```python
from build123d import *

# Parameters (mm, degrees)
F1_DEPTH = 63.5
F0_W     = 25.4
F0_H     = 19.05
F2_DEPTH = 25.4
F3_DEPTH = 7.9375
F5_R     = 6.35


with BuildPart() as f1:
    # F0 (on Front) → F1 (new body, symmetric)
    with BuildSketch(Plane.XZ):
        Polygon((-41.275, -9.525), (41.275, -9.525), (41.275, 9.525), (22.225, 9.525), (-41.275, 9.525), align=None)
    extrude(amount=F1_DEPTH, both=True)



with BuildPart() as f2:
    # F0 (on Front) → F2 (new body, symmetric)
    with BuildSketch(Plane.XZ):
        with BuildLine():
            Line((22.225, 9.525), (41.275, 9.525))
            Line((41.275, 9.525), (41.275, 26.9875))
            ThreePointArc((41.275, 26.9875), (45.9246798487, 38.2128201513), (57.15, 42.8625))
            Line((57.15, 42.8625), (60.325, 42.8625))
            Line((60.325, 42.8625), (60.325, 61.9125))
            Line((60.325, 61.9125), (57.15, 61.9125))
            add(Edge.make_bspline(
                [(56.2230819512, 61.9001975172), (56.5320743429, 61.9050863843), (56.8410510368, 61.9091866589), (57.15, 61.9125)],
                knots=[110.7034248849, 110.7034248849, 110.7034248849, 110.7034248849, 111.4985685166, 111.4985685166, 111.4985685166, 111.4985685166], degree=3))
            ThreePointArc((56.2230819512, 61.9001975172), (32.1287266725, 51.3532855624), (22.225, 26.9875))
            Line((22.225, 26.9875), (22.225, 9.525))
        make_face()
        with Locations((73.025, 52.3875)):
            Rectangle(F0_W, F0_H)
    extrude(amount=F2_DEPTH, both=True)


with BuildPart() as f1_1:
    add(f1.part)

    add(f2.part)  # F3 merges F2
    # F0 (on Front) → F3 (join, symmetric)
    with BuildSketch(Plane.XZ):
        with BuildLine():
            add(Edge.make_bspline(
                [(-41.275, 9.525), (-30.1197790598, 45.2532624962), (13.2037900148, 61.219547757), (56.2230819512, 61.9001975172)],
                knots=[0, 0, 0, 0, 110.7034248849, 110.7034248849, 110.7034248849, 110.7034248849], degree=3))
            Line((-41.275, 9.525), (22.225, 9.525))
            Line((22.225, 9.525), (22.225, 26.9875))
            ThreePointArc((22.225, 26.9875), (32.1287266725, 51.3532855624), (56.2230819512, 61.9001975172))
        make_face()
    extrude(amount=F3_DEPTH, both=True)

    # F0 (on Front) → F4 (revolve)
    with BuildSketch(Plane.XZ):
        Polygon((85.725, 61.9125), (85.725, 42.8625), (85.725, 38.1), (111.125, 38.1), (111.125, 66.675), (85.725, 66.675), align=None)
    revolve(axis=Axis((85.725, 0, 52.3875), (0, 0, 1)))

    # F5
    f5_edges = [f1_1.edges().sort_by_distance(p)[0] for p in [
        (-41.275, -63.5, 0),
        (41.275, -63.5, 0),
        (41.275, 63.5, 0),
        (-41.275, 63.5, 0),
    ]]
    fillet(f5_edges, radius=F5_R)


solid = f1_1.part
```
Input: part model. Units: mm. Frame: model coordinates. A direction names the side the tool comes from. Coordinates: 2 decimals unless noted, no trailing zeros. Write each loop counter-clockwise with the first axis right and the second up, starting at its lowest first coordinate (ties: lowest second). Pieces come first, ordered by that corner, then holes. Notation, with made-up numbers: (-14.5, 31) -> (29.5, 31) arc R26 ccw to (29.5, 54) -> close; hole circle Ø1 at (-7, -34). An arc over 180 degrees is marked (long way). Answer as a JSON object with one key per item and string values.
1. Mould query, pull axis X, two halves, no side actions, for faces 4 (the face through (-1, -1, -9.525)), 5 (the face through (39.464, -61.59, 0.133)), 6 (the face through (22.225, -17, 18)), 7 (the face through (45.802, -0.356, 38.089)). Classes: released by +X, released by -X, zero draft, split by the parting line, or undercut.
Result set:
{"face 4": "zero draft", "face 5": "released by +X", "face 6": "released by -X", "face 7": "undercut"}
2. First-contact query: P1, Ø5, axis at y = 14, z = 14, coming from the -X side (3 decimals); P2, Ø23, axis at x = 72.5, y = -11, coming from the -Z side; P3, Ø1, axis at y = -11.5, z = 51, coming from the -X side. Flat tips, straight axial feed; report the tip coordinate or a pass-through.
Result set:
{"P1": "stops at x = 22.225", "P2": "stops at z = 38.1", "P3": "stops at x = 31.33"}
3. Material intervals for line 1 (X direction, y = 29, z = 5) (3 decimals); line 2 (Z direction, x = 10, y = -50) (3 decimals); line 3 (Y direction, x = 79.5, z = 60.5), sorted ascending. Write a range as from..to.
Result set:
{"line 1": "x = -41.275..41.275", "line 2": "z = -9.525..9.525", "line 3": "y = -25.4..25.4"}
4. Access query for faces 1 (the face through (-3, -7.938, 30)), 2 (the face through (46, 25.4, 42)), 3 (the face through (-3, 7.938, 30)). Directions: +Z, -Z, +X, -X, +Y, -Y. A direction counts if a zero-diameter tool reaches every point of the face in a straight line with its end or side. Return the directions, or none.
Result set:
{"face 1": "+Z, -X, -Y", "face 2": "+Z, +X, -X, +Y", "face 3": "+Z, -X, +Y"}
5. Section A-A on y = 28. Return the cut outline in (x, z) (3 decimals), then the cut area to 3 significant figures.
Result set:
{"outline": "(-41.275, -9.525) -> (41.275, -9.525) -> (41.275, 9.525) -> (-41.275, 9.525) -> close", "area": "1,570 mm2"}
